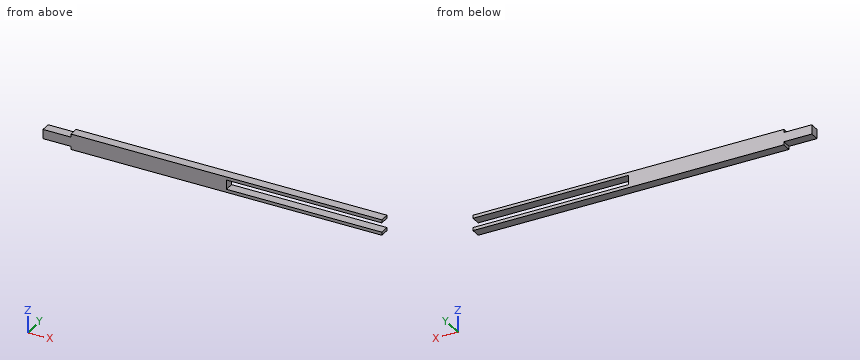
from build123d import *

# Parameters (mm, degrees)
SKETCH1_W           = 100
SKETCH1_H           = 5
BOSS_EXTRUDE1_DEPTH = 3
SKETCH2_W           = 50
SKETCH2_H           = 3.01
CUT_EXTRUDE1_DEPTH  = 3
SKETCH3_W           = 18
SKETCH3_H           = 3
BOSS_EXTRUDE2_DEPTH = 3


with BuildPart() as part:
    # Sketch1 → Boss-Extrude1 (new body)
    with BuildSketch(Plane(origin=(0, 0, 0), x_dir=(1, 0, 0), z_dir=(0, 1, 0))):
        Rectangle(SKETCH1_W, SKETCH1_H)
    extrude(amount=BOSS_EXTRUDE1_DEPTH)

    # Sketch2 → Cut-Extrude1 (cut)
    with BuildSketch(Plane(origin=(0, 3, 0), x_dir=(1, 0, 0), z_dir=(0, 1, 0))):
        with Locations((25, 0)):
            Rectangle(SKETCH2_W, SKETCH2_H)
    extrude(amount=-CUT_EXTRUDE1_DEPTH, mode=Mode.SUBTRACT)

    # Sketch3 → Boss-Extrude2 (add)
    with BuildSketch(Plane(origin=(0, 3, 0), x_dir=(1, 0, 0), z_dir=(0, 1, 0))):
        with Locations((-50, 0)):
            Rectangle(SKETCH3_W, SKETCH3_H)
    extrude(amount=-BOSS_EXTRUDE2_DEPTH)


solid = part.part
Work out the finished part from the listing and answer in its coordinate system (mm). Give positions to 0.01 mm unless a question says otherwise; leave off trailing zeros. Write each loop counter-clockwise with the first axis right and the second up, starting at its lowest first coordinate (ties: lowest second). Pieces come first, ordered by that corner, then holes.
Q1. The part is cut by section C-C on z = -0.55. Give the vertices of the cut face in (x, y), and give its area (3 significant figures).
Answer:
outline: (-59, 0) - (0, 0) - (0, 3) - (-59, 3) - close
area: 177 mm2
Q2. The part is cut by section A-A on x = 39.5. Give the vertices of the cut face in (y, z) (3 decimals), and give its area (3 significant figures).
Answer:
outline: (0, -2.5) - (3, -2.5) - (3, -1.505) - (0, -1.505) - close; (0, 1.505) - (3, 1.505) - (3, 2.5) - (0, 2.5) - close
area: 5.97 mm2
Q3. Given pin 1 (0.5 mm diameter, centred on y = 2, z = -2, fed in from -X), flat-ended and moving along its own axis, determine where the tip first touches the part or whether it passes through.
Answer:
pin 1: stops at x = -50
Q4. The part is cut by section B-B on y = 1.2. Give the vertices of the cut face in (x, z) (3 decimals).
Answer:
outline: (-59, -1.5) - (-50, -1.5) - (-50, -2.5) - (50, -2.5) - (50, -1.505) - (0, -1.505) - (0, 1.505) - (50, 1.505) - (50, 2.5) - (-50, 2.5) - (-50, 1.5) - (-59, 1.5) - close
Q5. Straight lines are drawn through the part: L1, parallel to Z at x = 23, y = 1.7 (3 decimals); L2, parallel to X at y = 2.1, z = -2; L3, parallel to X at y = 1.5, z = 1.4. For each, find the intervals that lie inside material, in ascending order.
Answer:
L1: z = -2.5 to -1.505, 1.505 to 2.5
L2: x = -50 to 50
L3: x = -59 to 0
